Geometry: final body of the model. Coordinates: model frame, mm. Face numbers are marked on the shaded views. A direction names the side the tool comes from. Coordinates: 2 decimals unless noted, no trailing zeros. Loops run counter-clockwise (first coordinate to the right, second up) from the corner with the lowest first, then second, coordinate; pieces in that order, holes last. Notation, with made-up numbers: (12, -32) - (46, -32) arc R25 cw to (46, 6) - close; hole circle Ø7 at (5, 30.5). An arc over 180 degrees is marked (long way). Put each result on its own line as item: value. Start each with the question number.
1) Section A-A on y = 38. Count the separate pieces of the cut face and the enclosed holes in it, and give its area (3 significant figures).
2) Section B-B on x = -245.5. Output: boundary loops of the cut face in (y, z) (1 decimal), and give its area (3 significant figures).
3) Section D-D on x = 194.5. Output: boundary loops of the cut face in (y, z) (1 decimal), and give its area (3 significant figures).
4) Draft query along Y for the marked faces 1 and 2. Return one class per face: +Y half, -Y half, draft (parallel to the pull), parting line (faces both ways), or undercut.
5) Reachability of the marked faces 3 and 4 from +Z, -Z, +X, -X, +Y, -Y: full face, straight path, thin tool, end or side. Return the list, or none.
6) Material intervals for line 1 along Y through (x, z) = (425, -44); line 2 along X through (y, z) = (-123.5, -36) (3 decimals); line 3 along Z through (x, y) = (-198.5, 98), sorted ascending. Write a range as from..to.
7) Section C-C on z = 27. Output: boundary loops of the cut face in (x, y) (3 decimals), and give its area (3 significant figures).
8) Contact query for flat-ended pins moving along their axis: pin 1 Ø12 at (y, z) = (-104, 6) entering from +X (3 decimals); pin 2 Ø10 at (x, y) = (425.45, -279.4) entering from -Z; pin 3 Ø8 at (x, z) = (-323, 3) entering from +Y (3 decimals). Output: stop coordinate, or through.
```python
from build123d import *

# Parameters (mm, degrees)
F4_DEPTH = 558.8
F5_R     = 6.35
F6_DEPTH = 92.076


with BuildPart() as f2:
    # F2: sweep along a path in F0
    with BuildLine(Plane.XY) as f2_path:
        Line((406.4, 279.4), (-406.4, 279.4))
        Line((-406.4, 279.4), (-406.4, -279.4))
        Line((-406.4, -279.4), (406.4, -279.4))
        Line((406.4, -279.4), (406.4, 279.4))
    # F1 (on Front) → F2 (sweep)
    with BuildSketch(Plane.XZ):
        Polygon((406.4, 46.0375), (406.4, 0), (406.4, -46.0375), (457.2, -46.0375), (457.2, -42.8625), (409.575, -42.8625), (409.575, 42.8625), (457.2, 42.8625), (457.2, 46.0375), align=None)
    sweep(path=f2_path.line, transition=Transition.RIGHT)

    # F3 (on face) → F4 (join, through all)
    with BuildSketch(Plane.XZ.offset(-279.4)):
        Polygon((-165.1, 46.0375), (-215.9, 46.0375), (-215.9, 42.8625), (-168.275, 42.8625), (-168.275, -42.8625), (-215.9, -42.8625), (-215.9, -46.0375), (-165.1, -46.0375), align=None)
        Polygon((165.1, -46.0375), (215.9, -46.0375), (215.9, -42.8625), (168.275, -42.8625), (168.275, 42.8625), (215.9, 42.8625), (215.9, 46.0375), (165.1, 46.0375), align=None)
    extrude(amount=F4_DEPTH)

    # F5 (on face) → F6 (cut, through all)
    with BuildSketch(Plane.XY.offset(46.0375)):
        with Locations((-425.45, -279.4)):
            Circle(F5_R)
        with Locations((-425.45, -31.75)):
            Circle(F5_R)
        with Locations((425.45, -279.4)):
            Circle(F5_R)
        with Locations((425.45, -31.75)):
            Circle(F5_R)
    extrude(amount=-F6_DEPTH, mode=Mode.SUBTRACT)


solid = f2.part
```
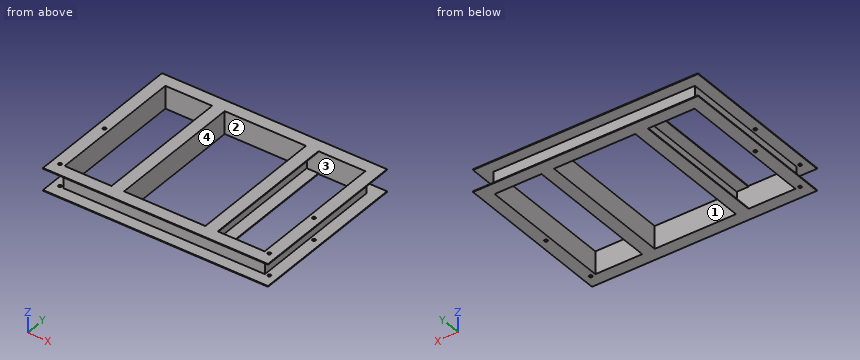
Answer block:
1. separate pieces: 4
1. enclosed holes: 0
1. area: 2,380 mm²
2. outline: (-330.2, -46) - (-279.4, -46) - (-279.4, 46) - (-330.2, 46) - (-330.2, 42.9) - (-282.6, 42.9) - (-282.6, -42.9) - (-330.2, -42.9) - close; (279.4, -46) - (330.2, -46) - (330.2, -42.9) - (282.6, -42.9) - (282.6, 42.9) - (330.2, 42.9) - (330.2, 46) - (279.4, 46) - close
2. area: 1,190 mm²
3. outline: (-330.2, -46) - (330.2, -46) - (330.2, -42.9) - (282.6, -42.9) - (282.6, 42.9) - (330.2, 42.9) - (330.2, 46) - (-330.2, 46) - (-330.2, 42.9) - (-282.6, 42.9) - (-282.6, -42.9) - (-330.2, -42.9) - close; hole (-279.4, -42.9) - (279.4, -42.9) - (279.4, 42.9) - (-279.4, 42.9) - close
3. area: 4,740 mm²
4. face 1: undercut
4. face 2: undercut
5. face 3: none
5. face 4: +Z, -Z
6. line 1: y = -330.2..-285.73, -273.07..-38.08, -25.42..330.2
6. line 2: x = -409.575..-406.4, -168.275..-165.1, 165.1..168.275, 406.4..409.575
6. line 3: z = -46.04..-42.86, 42.86..46.04
7. outline: (-409.575, -282.575) - (409.575, -282.575) - (409.575, 282.575) - (-409.575, 282.575) - close; hole (-406.4, -279.4) - (-168.275, -279.4) - (-168.275, 279.4) - (-406.4, 279.4) - close; hole (-165.1, -279.4) - (165.1, -279.4) - (165.1, 279.4) - (-165.1, 279.4) - close; hole (168.275, -279.4) - (406.4, -279.4) - (406.4, 279.4) - (168.275, 279.4) - close
7. area: 12,300 mm²
8. pin 1: stops at x = 409.575
8. pin 2: passes through
8. pin 3: stops at y = 282.575
